Design review of the part built by this model. Coordinates are the model's own, in mm. Face numbers are marked on the shaded views. A direction names the side the tool comes from. Coordinates: 2 decimals unless noted, no trailing zeros. Loops run counter-clockwise (first coordinate to the right, second up) from the corner with the lowest first, then second, coordinate; pieces in that order, holes last. Notation, with made-up numbers: (39, 24.5) - (74, 24.5) arc R31 cw to (74, 48.5) - close; hole circle Ø6 at (-38, 34). An arc over 180 degrees is marked (long way). Return JSON: item names as keys, results as strings. Group by question number.
from build123d import *

# Parameters (mm, degrees)
F0_W     = 42.7631036925
F0_H     = 22.0432821037
F0_H_2   = 7.9567178963
F0_H_3   = 20
F1_DEPTH = 12.5
F2_R     = 11.5788396241
F3_DEPTH = 50
F4_R     = 16.9293792231
F5_DEPTH = 47.1764579415


with BuildPart() as f1:
    # F0 (on Front) → F1 (new body, symmetric)
    with BuildSketch(Plane.XZ):
        Polygon((25, 30), (-45, 30), (-45, -30), (45, -30), (45, 30), align=None)
        with BuildLine():
            add(Edge.make_bspline(
                [(-45, 30), (-49.6783256531, 98.533667624), (19.1648956388, 126.3746768236), (65, 102.0432821037)],
                knots=[0, 0, 0, 0, 131.4923362644, 131.4923362644, 131.4923362644, 131.4923362644], degree=3))
            Line((-45, 30), (25, 30))
            Line((25, 30), (25, 62.0432821037))
            ThreePointArc((25, 62.0432821037), (36.7157287525, 90.3275533511), (65, 102.0432821037))
        make_face()
        with Locations((97.3985187706, 71.0216410518)):
            Rectangle(F0_W, F0_H)
        with Locations((97.3985187706, 106.0216410518)):
            Rectangle(F0_W, F0_H_2)
        with BuildLine():
            Line((25, 62.0432821037), (25, 30))
            Line((25, 30), (45, 30))
            Line((45, 30), (45, 62.0432821037))
            ThreePointArc((45, 62.0432821037), (50.8578643763, 76.1854177274), (65, 82.0432821037))
            Line((65, 82.0432821037), (76.0169669243, 82.0432821037))
            Line((76.0169669243, 82.0432821037), (76.0169669243, 102.0432821037))
            Line((76.0169669243, 102.0432821037), (65, 102.0432821037))
            ThreePointArc((65, 102.0432821037), (36.7157287525, 90.3275533511), (25, 62.0432821037))
        make_face()
        Polygon((118.7800706168, 110), (118.7800706168, 102.0432821037), (118.7800706168, 82.0432821037), (118.7800706168, 60), (145.7395272495, 60), (145.7395272495, 110), align=None)
        with Locations((97.3985187706, 92.0432821037)):
            Rectangle(F0_W, F0_H_3)
    extrude(amount=F1_DEPTH, both=True)

    # F2 (on face) → F3 (join)
    with BuildSketch(Plane.XY.offset(110)):
        with Locations((145.7395272495, 0)):
            Circle(F2_R)
    extrude(amount=-F3_DEPTH)

    # F4 (on face) → F5 (join)
    with BuildSketch(Plane.XZ.offset(12.5)):
        with Locations((107.2820425034, 81.4744457603)):
            Circle(F4_R)
    extrude(amount=F5_DEPTH)


solid = f1.part
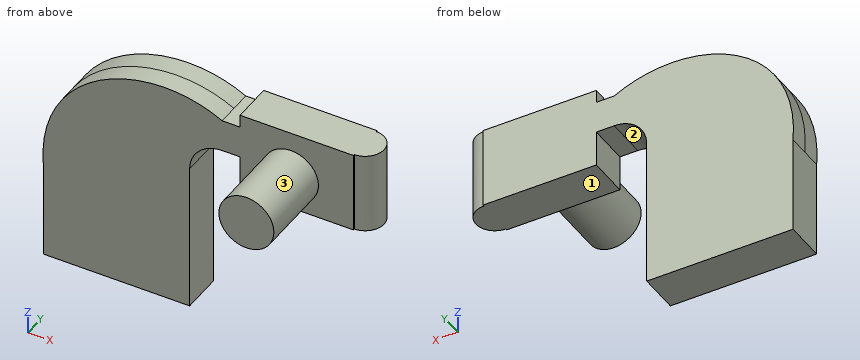
Item 1: For P1, Ø12.5, axis at x = 129.5, y = 2.5, coming from the +Z side; P2, Ø2, axis at x = 73.5, y = -6, coming from the +Z side; P3, Ø20, axis at y = 6, z = -12, coming from the -X side, all flat-tipped, find the tip position at first contact; note any pin that passes through.
Item 2: Add section B-B (z = 4). State the section outline as (x, y) points.
Item 3: For the marked faces 1, 2 and 3, list the 3-axis set-ups (+Z, -Z, +X, -X, +Y, -Y) from which the entire face can be reached by the end or side of a thin tool; tool diameter is ignored.
Item 4: To check wall thickness, follow line 1 (Y direction, x = -1, z = 95.5); line 2 (Z direction, x = 78.5, y = 1.5); line 3 (X direction, y = 0.5, z = -21). State the ranges of each line that lie inside material, in increasing order. Write a range as from..to.
Item 5: Add section A-A (x = 133). State the section outline as (y, z) points.
Answers below:
{
 "1": {"P1": "stops at z = 110", "P2": "stops at z = 102.04", "P3": "stops at x = -45"},
 "2": {"outline": "(-45, -12.5) - (45, -12.5) - (45, 12.5) - (-45, 12.5) - close"},
 "3": {"face 1": "-Z, +X, +Y, -Y", "face 2": "-Z, +Y, -Y", "face 3": "-Y"},
 "4": {"line 1": "y = -12.5..12.5", "line 2": "z = 60..110", "line 3": "x = -45..45"},
 "5": {"outline": "(-12.5, 60) - (12.5, 60) - (12.5, 110) - (-12.5, 110) - close"}
}
